Answer from the drawing. Dimensions are ordinates in mm from the lowest x, y and z of the part. A direction names the side the tool comes from. Coordinates: 2 decimals unless noted, no trailing zeros. Order: outer loops, then holes, each group sorted by start corner. A loop starts at its lowest first (then second) coordinate and runs counter-clockwise, first axis right, second up. Notation, with made-up numbers: (62.5, -30) - (81.5, -30) arc R15 cw to (81.5, -18) - close; hole circle Ø2 at (-9, -35). An arc over 180 degrees is marked (long way). Answer as a JSON object with one key per item and string values. Group by question number.
1) Each of these flat-tipped pins is pushed along its axis until it touches: P1, Ø4, axis at x = 14, z = 37.5, coming from the +Y side; P2, Ø13.5, axis at x = 17.5, z = 61.5, coming from the +Y side; P3, Ø8, axis at x = 22.5, z = 73.5, coming from the -Y side. Where does it stop, or does it pass through?
2) Section A-A (x = 13.5) is taken. Give the vertices of the cut face in (y, z) (3 decimals), plus the area to 3 significant figures.
3) A tool of negligible diameter and unlimited length cuts with its end or side. For the marked faces 1, 2 and 3, from which of +Z, -Z, +X, -X, +Y, -Y can it reach the whole face along a straight path? Write none if from no direction.
4) Section D-D (z = 68.5) is taken. Give the vertices of the cut face in (x, y).
5) The mould has two halves that part along Y. Classify the marked faces 4, 5 and 6: released by +Y, released by -Y, zero draft, split by the parting line, or undercut.
6) Section B-B (y = 4.5) is taken. Give the vertices of the cut face in (x, z), plus the area to 3 significant figures.
7) Section C-C (z = 42) is taken. Give the vertices of the cut face in (x, y), plus the area to 3 significant figures.
8) Find the intervals of material crossed by line 1 along Y through (x, z) = (37, 42); line 2 along Z through (x, y) = (23.5, 33.5); line 3 along Z through (x, y) = (14, 39) (3 decimals), in increasing order.
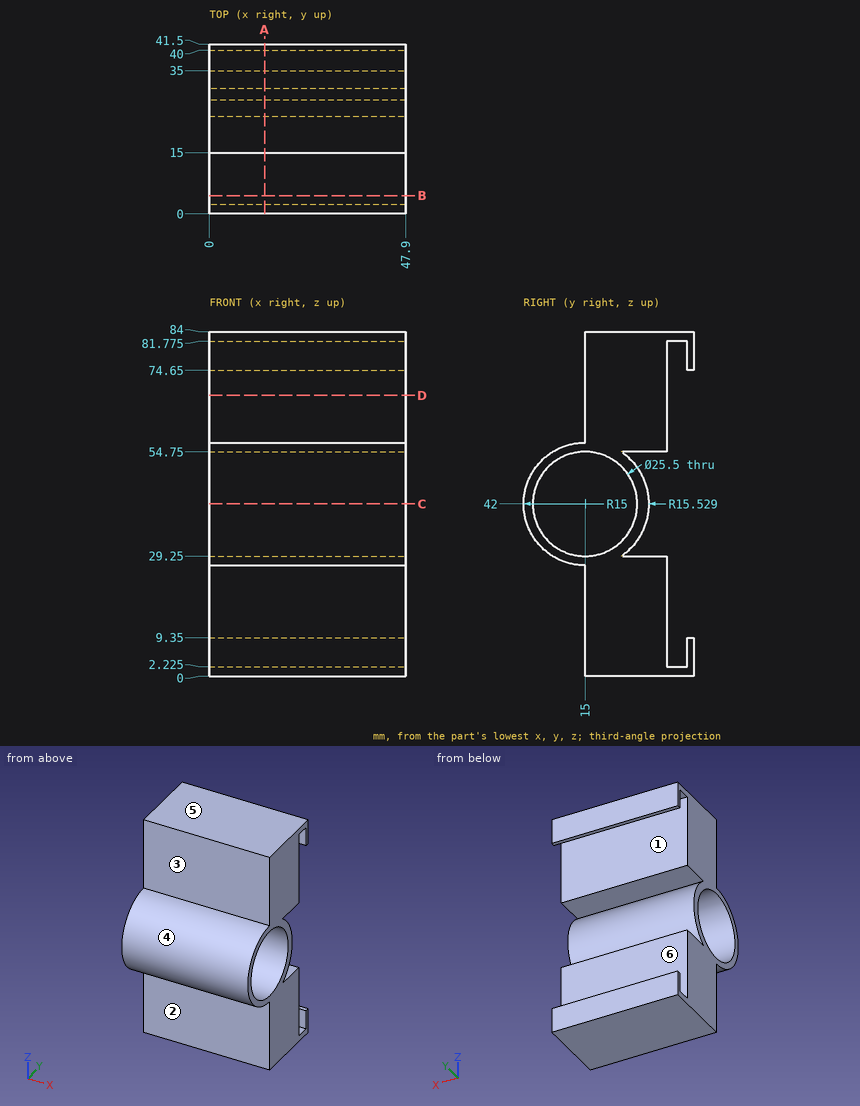
Report:
{
 "1": {"P1": "stops at y = 30.33", "P2": "stops at y = 35", "P3": "stops at y = 15"},
 "2": {"outline": "(15, 0) - (41.5, 0) - (41.5, 9.35) - (40, 9.35) - (40, 2.225) - (35, 2.225) - (35, 29.25) - (23.865, 29.25) arc R15.529 ccw to (23.865, 54.75) - (35, 54.75) - (35, 81.775) - (40, 81.775) - (40, 74.65) - (41.5, 74.65) - (41.5, 84) - (15, 84) - (15, 57) arc R15 ccw to (15, 27) - close; hole circle Ø25.5 at (15, 42)", "area": "1,410 mm²"},
 "3": {"face 1": "+X, -X", "face 2": "-Z, +X, -X, -Y", "face 3": "+Z, +X, -X, -Y"},
 "4": {"outline": "(0, 15) - (47.9, 15) - (47.9, 35) - (0, 35) - close"},
 "5": {"face 4": "released by -Y", "face 5": "zero draft", "face 6": "undercut"},
 "6": {"outline": "(0, 31.29) - (47.9, 31.29) - (47.9, 34.77) - (0, 34.77) - close; (0, 49.23) - (47.9, 49.23) - (47.9, 52.71) - (0, 52.71) - close", "area": "333 mm²"},
 "7": {"outline": "(0, 0) - (47.9, 0) - (47.9, 2.25) - (0, 2.25) - close; (0, 27.75) - (47.9, 27.75) - (47.9, 30.53) - (0, 30.53) - close", "area": "241 mm²"},
 "8": {"line 1": "y = 0 to 2.25, 27.75 to 30.53", "line 2": "z = 0 to 29.25, 54.75 to 84", "line 3": "z = 0 to 2.225, 81.775 to 84"}
}
